Geometry check sheet. Reference: the model listing, model coordinates, mm. A direction names the side the tool comes from. Give positions to 0.01 mm unless a question says otherwise; leave off trailing zeros. Order: outer loops, then holes, each group sorted by start corner. A loop starts at its lowest first (then second) coordinate and runs counter-clockwise, first axis right, second up. Notation, with made-up numbers: M 56.25,89.25 L 96.25,89.25 A23 ccw 96.25,126.25 Z; hole C 7.5,14 d8. An arc over 180 degrees is marked long. Answer as CSV lines item,"result". Start each with the question number.
Q1. Go/stop test with flat-tipped pins: pin 1 (2 mm diameter, centred on x = 16.5, z = 0.5, fed in from +Y); pin 2 (2 mm diameter, centred on x = 10, z = 2, fed in from +Y); pin 3 (5 mm diameter, centred on x = 5, z = 3, fed in from +Y). Record where each tip stops, or that it passes through.
Q2. Thickness scan on line 1 (Z direction, x = 8, y = 0); line 2 (Z direction, x = 11.5, y = -2); line 3 (X direction, y = 3, z = -1.25). Record the ranges inside material, lowest first.
Q3. Set-up check for faces 4 (the flat face through (25, 2, -2)), 5 (the flat face through (29, -2, 0)), 6 (the flat face through (27, -1.25, 0)): record each of +Z, -Z, +X, -X, +Y, -Y from which the full face is reachable in a straight line by a thin tool's end or side.
Q4. Mould release check, pull along Y, two halves, no side actions. Record for faces 1 (the cylindrical face through (26.73, -0.59, 4.46)), 2 (the flat face through (27.03, -0.63, -1.08)), 3 (the flat face through (0, 0, 0)): +Y half, -Y half, draft (parallel to the pull), parting line (faces both ways), or undercut.
Q5. Section check A-A, the plane x = 22.5. Record the boundary of the cut face in (y, z), then the cut area to 3 significant figures.
```python
from build123d import *

# Parameters (mm, degrees)
CUT_EXTRUDE1_DEPTH = 4


with BuildPart() as part:
    # Sketch1 → Revolve1 (revolve)
    with BuildSketch(Plane.XY):
        Polygon((0, 0), (29, 0), (29, 4), (28.5, 4.5), (25, 4.5), (25, 2.5), (5, 2.5), (5, 2), (0.5, 2), (0, 1.5), align=None)
    revolve(axis=Axis((0, 0, 0), (1, 0, 0)))

    # Sketch2 → Cut-Extrude1 (cut)
    with BuildSketch(Plane(origin=(29, 0, 0), x_dir=(0, 0, -1), z_dir=(1, 0, 0))):
        Polygon((1.443375673, 0), (0.721687836, 1.25), (-0.721687836, 1.25), (-1.443375673, 0), (-0.721687836, -1.25), (0.721687836, -1.25), align=None)
    extrude(amount=-CUT_EXTRUDE1_DEPTH, mode=Mode.SUBTRACT)


solid = part.part
```
Answer block:
1,pin 1,"stops at y = 2.5"
1,pin 2,"stops at y = 2.29"
1,pin 3,"stops at y = 2.45"
2,line 1,"z = -2.5 to 2.5"
2,line 2,"z = -1.5 to 1.5"
2,line 3,"x = 25 to 29"
3,face 4,"-X"
3,face 5,"+Z, -Z, +X, +Y, -Y"
3,face 6,"+X"
4,face 1,"parting line"
4,face 2,"undercut"
4,face 3,"draft"
5,outline,"C 0,0 d5"
5,area,"19.6 mm2"
